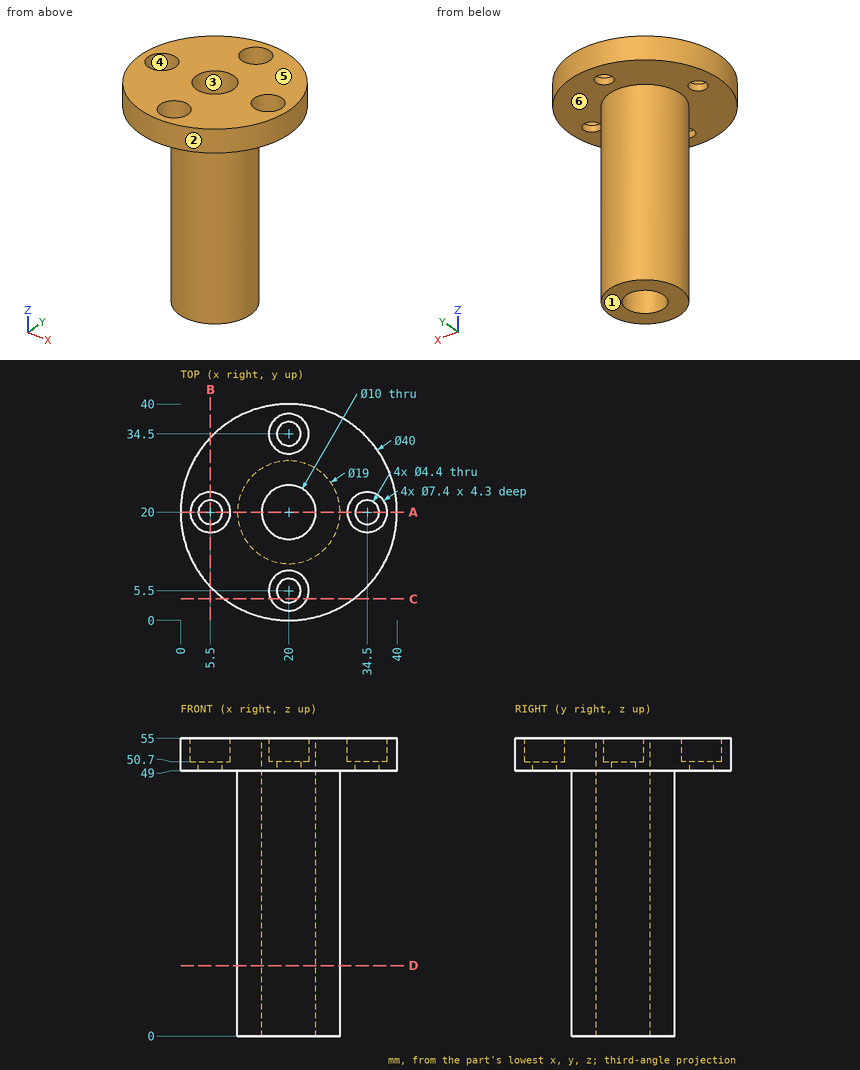
Design review of the part shown in the three views and the two pictorial views. Dimensions are in mm from the part's minimum x, y and z. A direction names the side the tool comes from. Give positions to 0.01 mm unless a question says otherwise; leave off trailing zeros. Loops run counter-clockwise (first coordinate to the right, second up) from the corner with the lowest first, then second, coordinate; pieces in that order, holes last. Notation, with made-up numbers: M 59,77 L 68,77 A17 ccw 68,89 Z; hole C 4,31.25 d5. An arc over 180 degrees is marked long. Answer as a JSON object with one key per item and string values. Group by question number.
Q1. Tool access review of the marked faces 4, 5 and 6: name each direction out of +Z, -Z, +X, -X, +Y, -Y from which nothing blocks a thin tool from reaching the whole face with its end or side.
Q2. Insertion check: P1, Ø7, axis at x = 34.5, y = 20, coming from the -Z side; P2, Ø1, axis at x = 18.5, z = 43, coming from the +Y side; P3, Ø5.5, axis at x = 20, y = 34.5, coming from the +Z side. Each pin has a flat end and moves straight along its axis. Give the tip position at first contact, or say it passes through.
Q3. Mouldability with a two-part tool opening along X and no side actions: class the marked faces 1, 2 and 3 as +X half, -X half, draft (parallel to the pull), parting line (faces both ways), or undercut.
Q4. Add section D-D on z = 13. Give the boundary of the cut face in (x, y), and give its area (3 significant figures).
Q5. Add section A-A on y = 20. Give the boundary of the cut face in (x, z).
Q6. Add section C-C on y = 4. Give the boundary of the cut face in (x, z), and give its area (3 significant figures).
Q7. For probe 1 along X at (y, z) = (20, 52.1); probe 2 along X at (y, z) = (20, 49.9), list the stretches that pass through material, from the lowest coordinate up. Write a range as [from, to].
Q8. Add section B-B on x = 5.5. Give the boundary of the cut face in (y, z), and give its area (3 significant figures).
Checked values:
{
 "1": {"face 4": "+Z", "face 5": "+Z, +X, -X, +Y, -Y", "face 6": "-Z"},
 "2": {"P1": "z = 49", "P2": "y = 29.45", "P3": "z = 50.7"},
 "3": {"face 1": "draft", "face 2": "parting line", "face 3": "undercut"},
 "4": {"outline": "C 20,20 d19; hole C 20,20 d10", "area": "205 mm²"},
 "5": {"outline": "M 0,49 L 3.3,49 L 3.3,50.7 L 1.8,50.7 L 1.8,55 L 0,55 Z; M 7.7,49 L 10.5,49 L 10.5,0 L 15,0 L 15,55 L 9.2,55 L 9.2,50.7 L 7.7,50.7 Z; M 25,0 L 29.5,0 L 29.5,49 L 32.3,49 L 32.3,50.7 L 30.8,50.7 L 30.8,55 L 25,55 Z; M 36.7,49 L 40,49 L 40,55 L 38.2,55 L 38.2,50.7 L 36.7,50.7 Z"},
 "6": {"outline": "M 8,49 L 18.39,49 L 18.39,50.7 L 16.62,50.7 L 16.62,55 L 8,55 Z; M 21.61,49 L 32,49 L 32,55 L 23.38,55 L 23.38,50.7 L 21.61,50.7 Z", "area": "109 mm²"},
 "7": {"probe 1": "[0, 1.8], [9.2, 15], [25, 30.8], [38.2, 40]", "probe 2": "[0, 3.3], [7.7, 15], [25, 32.3], [36.7, 40]"},
 "8": {"outline": "M 6.23,49 L 17.8,49 L 17.8,50.7 L 16.3,50.7 L 16.3,55 L 6.23,55 Z; M 22.2,49 L 33.77,49 L 33.77,55 L 23.7,55 L 23.7,50.7 L 22.2,50.7 Z", "area": "126 mm²"}
}
